Read the model definition and answer for the solid it produces. Units are mm, in the model's axes. A direction names the side the tool comes from. Coordinates: 2 decimals unless noted, no trailing zeros. Order: outer loops, then holes, each group sorted by start corner. A loop starts at its lowest first (then second) coordinate and runs counter-clockwise, first axis right, second up. Notation, with made-up numbers: M 52,79.25 L 73,79.25 A18 cw 73,84.25 Z; hole C -25.5,-23.75 d8. An arc over 180 degrees is marked long. Use a Markdown table: item, result. Add a question column.
1) Find the intervals of material crossed by probe 1 along Y at (x, z) = (30, 41); probe 2 along X at (y, z) = (-9.5, 12.5) (3 decimals); probe 3 along Z at (x, y) = (-29, 37.5) (3 decimals), in increasing order. Write a range as [from, to].
2) For faces 5 (the face through (-4, -7.938, 30)), 6 (the face through (61, -20, 42.809)), 7 (the face through (-4, 7.938, 30)), 8 (the face through (105.322, 7.659, 52.579)), determine the directions among +Z, -Z, +X, -X, +Y, -Y from which every point of the face is accessible in a straight line to the end or side of a thin tool.
3) Find section B-B on y = 48.5. Write down the section's boundary in (x, z) (3 decimals), plus the area to 3 significant figures.
4) Find section A-A on z = 5. Write down the section's boundary in (x, y) (3 decimals), plus the area to 3 significant figures.
5) The mould has two halves that part along X. Classify faces 1 (the face through (61, 21, 61.895)), 2 (the face through (32.21, 16.55, 51.45)), 3 (the face through (61, 20, 42.809)), 4 (the face through (39.464, 61.59, 0.133)): released by +X, released by -X, zero draft, split by the parting line, or undercut.
6) Each of these flat-tipped pins is pushed along its axis until it touches: pin 1 Ø6 at (y, z) = (37.5, 10) entering from +X (3 decimals); pin 2 Ø4 at (x, y) = (1, 30.5) entering from +Z (3 decimals); pin 3 Ø8.5 at (x, y) = (62, 17) entering from +Z. Where does it stop, or does it pass through?
from build123d import *

# Parameters (mm, degrees)
F1_DEPTH = 63.5
F2_DEPTH = 25.4
F3_DEPTH = 7.9375
F4_DEPTH = 25.4
F6_R     = 6.35


with BuildPart() as f1:
    # F0 (on Front) → F1 (new body, symmetric)
    with BuildSketch(Plane.XZ):
        Polygon((22.225, 9.525), (-41.275, 9.525), (-41.275, -9.525), (41.275, -9.525), (41.275, 9.525), align=None)
    extrude(amount=F1_DEPTH, both=True)

    # F0 (on Front) → F2 (join, symmetric)
    with BuildSketch(Plane.XZ):
        with BuildLine():
            Line((22.225, 27.0002), (22.225, 9.525))
            Line((22.225, 9.525), (41.275, 9.525))
            Line((41.275, 9.525), (41.275, 27.0002))
            ThreePointArc((41.275, 27.0002), (45.4231719771, 37.70053315), (55.6998352153, 42.8088257182))
            Line((55.6998352153, 42.8088257182), (55.6998352153, 61.8950799553))
            ThreePointArc((55.6998352153, 61.8950799553), (31.9467995078, 51.1777579815), (22.225, 27.0002))
        make_face()
    extrude(amount=F2_DEPTH, both=True)

    # F0 (on Front) → F3 (join, symmetric)
    with BuildSketch(Plane.XZ):
        with BuildLine():
            add(Edge.make_bspline(
                [(-41.275, 9.525), (-40.1314669034, 30.5728232182), (15.8217890978, 61.4964285617), (55.6998352153, 61.9232521068)],
                knots=[0, 0, 0, 0, 110.1624749452, 110.1624749452, 110.1624749452, 110.1624749452], degree=3))
            Line((-41.275, 9.525), (22.225, 9.525))
            Line((22.225, 9.525), (22.225, 27.0002))
            ThreePointArc((22.225, 27.0002), (31.9467995078, 51.1777579815), (55.6998352153, 61.8950799553))
            Line((55.6998352153, 61.8950799553), (55.6998352153, 61.9232521068))
        make_face()
    extrude(amount=F3_DEPTH, both=True)

    # F4 (add): a face of the model
    f4_faces = [f1.faces().sort_by_distance(p)[0] for p in [
        (55.6998352153, 0, 52.3563592003),
    ]]
    extrude(f4_faces, amount=F4_DEPTH)

    # F0 (on Front) → F5 (revolve)
    with BuildSketch(Plane.XZ):
        Polygon((106.4998352153, 66.675), (80.9040206471, 66.675), (81.0998352153, 38.1), (106.4998352153, 38.1), align=None)
    revolve(axis=Axis((81.0019279312, 0, 52.3875), (-0.0068524924, 0, 0.9999765214)))

    # F6
    f6_edges = [f1.edges().sort_by_distance(p)[0] for p in [
        (-41.275, 63.5, 0),
        (-41.275, -63.5, 0),
        (41.275, -63.5, 0),
        (41.275, 63.5, 0),
    ]]
    fillet(f6_edges, radius=F6_R)


solid = f1.part
Check result:
| question | item | result |
|---|---|---|
| 1 | probe 1 | y = [-25.4, 25.4] |
| 1 | probe 2 | x = [22.225, 41.275] |
| 1 | probe 3 | z = [-9.525, 9.525] |
| 2 | face 5 | +Z, -X, -Y |
| 2 | face 6 | -Z, -Y |
| 2 | face 7 | +Z, -X, +Y |
| 2 | face 8 | none |
| 3 | outline | M -41.275,-9.525 L 41.275,-9.525 L 41.275,9.525 L -41.275,9.525 Z |
| 3 | area | 1,570 mm2 |
| 4 | outline | M -41.275,-57.15 A6.35 ccw -34.925,-63.5 L 34.925,-63.5 A6.35 ccw 41.275,-57.15 L 41.275,57.15 A6.35 ccw 34.925,63.5 L -34.925,63.5 A6.35 ccw -41.275,57.15 Z |
| 4 | area | 10,400 mm2 |
| 5 | face 1 | zero draft |
| 5 | face 2 | released by -X |
| 5 | face 3 | undercut |
| 5 | face 4 | released by +X |
| 6 | pin 1 | stops at x = 41.275 |
| 6 | pin 2 | stops at z = 9.525 |
| 6 | pin 3 | stops at z = 66.43 |
